```python
from build123d import *
from OCP.BRepFilletAPI import BRepFilletAPI_MakeChamfer

# Parameters (mm, degrees)
SKETCH1_W           = 22.5
SKETCH1_H           = 38
BOSS_EXTRUDE2_DEPTH = 7
SKETCH2_W           = 22.5
SKETCH2_H           = 38
BOSS_EXTRUDE4_DEPTH = 2.5
SKETCH3_W           = 12
SKETCH3_H           = 12
CUT_EXTRUDE1_DEPTH  = 2.5
CHAMFER1_SIZE       = 1.5
FILLET3_R           = 2
FILLET4_R           = 2
CHAMFER2_SIZE       = 3
CHAMFER2_SIZE2      = 1.732050808
FILLET5_R           = 2


with BuildPart() as part:
    # Sketch1 → Boss-Extrude2 (new body)
    with BuildSketch(Plane(origin=(0, 0, 0), x_dir=(1, 0, 0), z_dir=(0, 1, 0))):
        Rectangle(SKETCH1_W, SKETCH1_H)
        Polygon((-8.05, -15.8), (-8.05, -4.492937268), (-10.337901284, -4.492937268), (-10.337901284, 0), (-10.337901284, 4.511829369), (-8.05, 4.511829369), (-8.05, 15.8), (8.05, 15.8), (8.05, 4.494825775), (10.314669875, 4.494825775), (10.314669875, 0), (10.314669875, -4.426605317), (8.05, -4.426605317), (8.05, -15.8), align=None, mode=Mode.SUBTRACT)
    extrude(amount=BOSS_EXTRUDE2_DEPTH)

    # Sketch2 → Boss-Extrude4 (add)
    with BuildSketch(Plane(origin=(0, 7, 0), x_dir=(1, 0, 0), z_dir=(0, 1, 0))):
        Rectangle(SKETCH2_W, SKETCH2_H)
    extrude(amount=BOSS_EXTRUDE4_DEPTH)

    # Sketch3 → Cut-Extrude1 (cut)
    with BuildSketch(Plane(origin=(0, 9.5, 0), x_dir=(1, 0, 0), z_dir=(0, 1, 0))):
        Rectangle(SKETCH3_W, SKETCH3_H)
    extrude(amount=-CUT_EXTRUDE1_DEPTH, mode=Mode.SUBTRACT)

    # Chamfer1
    chamfer1_edges = [part.edges().sort_by_distance(p)[0] for p in [
        (6, 8.25, -6),
        (6, 8.25, 6),
        (-6, 8.25, 6),
        (-6, 8.25, -6),
    ]]
    chamfer(chamfer1_edges, length=CHAMFER1_SIZE)

    # Fillet3
    fillet3_edges = [part.edges().sort_by_distance(p)[0] for p in [
        (8.05, 7, 10.113302659),
        (0, 7, 15.8),
        (-8.05, 7, 10.146468634),
        (-9.193950642, 7, 4.492937268),
        (-8.05, 3.5, 15.8),
        (8.05, 3.5, 15.8),
        (-9.193950642, 7, -4.511829369),
        (-8.05, 7, -10.155914685),
        (0, 7, -15.8),
        (8.05, 7, -10.147412887),
        (9.182334937, 7, -4.494825775),
        (9.182334937, 7, 4.426605317),
    ]]
    fillet(fillet3_edges, radius=FILLET3_R)

    # Fillet4
    # the kernel refuses this fillet: 2 mm, written as the material it adds along each edge
    with BuildSketch(Plane(origin=(-6.05, 5, -13.8), x_dir=(-1, 0, 0), z_dir=(0, 0, -1))) as fillet4_piece_1_section:
        Polygon((0, 0), (FILLET4_R, 0), (FILLET4_R, FILLET4_R), (0, FILLET4_R), align=None)
    fillet4_piece_1 = extrude(amount=FILLET4_R, mode=Mode.PRIVATE)
    fillet4_piece_1 = fillet4_piece_1 - Plane(origin=(-6.05, 5, -13.8), x_dir=(0.7071067811865475, -0.7071067811865475, 0), z_dir=(0, 0, -1)) * Sphere(FILLET4_R, mode=Mode.PRIVATE)
    add(fillet4_piece_1)
    with BuildSketch(Plane(origin=(6.05, 5, -13.8), x_dir=(0, 0, -1), z_dir=(1, 0, 0))) as fillet4_piece_2_section:
        Polygon((0, 0), (FILLET4_R, 0), (FILLET4_R, FILLET4_R), (0, FILLET4_R), align=None)
    fillet4_piece_2 = extrude(amount=FILLET4_R, mode=Mode.PRIVATE)
    fillet4_piece_2 = fillet4_piece_2 - Plane(origin=(6.05, 5, -13.8), x_dir=(0, -0.7071067811865475, 0.7071067811865475), z_dir=(1, 0, 0)) * Sphere(FILLET4_R, mode=Mode.PRIVATE)
    add(fillet4_piece_2)
    with BuildSketch(Plane(origin=(8.05, 0, -15.8), x_dir=(0, 0, 1), z_dir=(0, 1, 0)), Plane(origin=(-8.05, 0, -15.8), x_dir=(1, 0, 0), z_dir=(0, 1, 0))) as fillet4_piece_3:
        with BuildLine():
            CenterArc((FILLET4_R, -FILLET4_R), FILLET4_R, 90, 90)
            Line((0, -FILLET4_R), (0, 0))
            Line((0, 0), (FILLET4_R, 0))
        make_face()
    extrude(amount=5)

    # Chamfer2: one chamfer whose edges measure the first distance from different faces: ONE call of the kernel's chamfer builder (chamfer() names one face for all edges)
    chamfer2_edges_1 = [part.edges().sort_by_distance(p)[0] for p in [
        (11.25, 9.5, 0),
    ]]
    chamfer2_side_1 = [part.faces().sort_by_distance(p)[0] for p in [
        (11.25, 4.75, 0),
    ]]
    chamfer2_edges_2 = [part.edges().sort_by_distance(p)[0] for p in [
        (0, 9.5, -19),
    ]]
    chamfer2_side_2 = [part.faces().sort_by_distance(p)[0] for p in [
        (0, 4.75, -19),
    ]]
    chamfer2_edges_3 = [part.edges().sort_by_distance(p)[0] for p in [
        (-11.25, 9.5, 0),
    ]]
    chamfer2_side_3 = [part.faces().sort_by_distance(p)[0] for p in [
        (-11.25, 4.75, 0),
    ]]
    chamfer2_edges_4 = [part.edges().sort_by_distance(p)[0] for p in [
        (0, 9.5, 19),
    ]]
    chamfer2_side_4 = [part.faces().sort_by_distance(p)[0] for p in [
        (0, 4.75, 19),
    ]]
    chamfer2 = BRepFilletAPI_MakeChamfer(part.part.solid().wrapped)
    for e in chamfer2_edges_1:
        chamfer2.Add(CHAMFER2_SIZE, CHAMFER2_SIZE2, e.wrapped, chamfer2_side_1[0].wrapped)  # the first distance lies on this face
    for e in chamfer2_edges_2:
        chamfer2.Add(CHAMFER2_SIZE, CHAMFER2_SIZE2, e.wrapped, chamfer2_side_2[0].wrapped)  # the first distance lies on this face
    for e in chamfer2_edges_3:
        chamfer2.Add(CHAMFER2_SIZE, CHAMFER2_SIZE2, e.wrapped, chamfer2_side_3[0].wrapped)  # the first distance lies on this face
    for e in chamfer2_edges_4:
        chamfer2.Add(CHAMFER2_SIZE, CHAMFER2_SIZE2, e.wrapped, chamfer2_side_4[0].wrapped)  # the first distance lies on this face
    add(Compound.cast(chamfer2.Shape()), mode=Mode.REPLACE)

    # Fillet5
    fillet5_edges = [part.edges().sort_by_distance(p)[0] for p in [
        (-11.25, 6.5, 0),
        (0, 6.5, -19),
        (11.25, 6.5, 0),
        (0, 6.5, 19),
    ]]
    fillet(fillet5_edges, radius=FILLET5_R)


solid = part.part
```
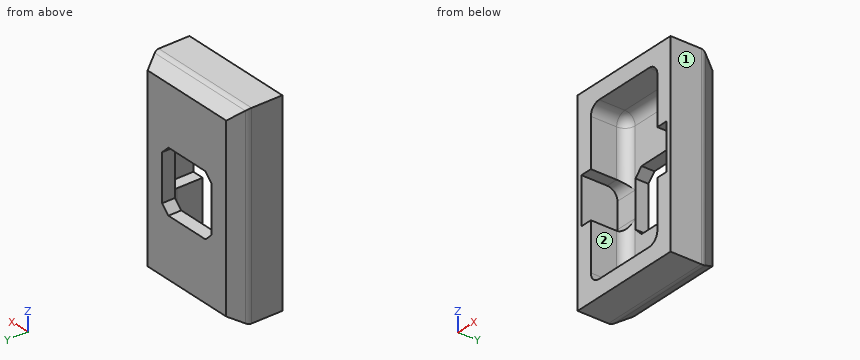
Model file for the job. Use its own axes, mm. Face numbers are marked on the shaded views. A direction names the side the tool comes from. Coordinates: 2 decimals unless noted, no trailing zeros. Write each loop counter-clockwise with the first axis right and the second up, starting at its lowest first coordinate (ties: lowest second). Pieces come first, ordered by that corner, then holes. Notation, with made-up numbers: (27.25, -14.75) - (74.25, -14.75) arc R17 cw to (74.25, -0.75) - close; hole circle Ø10 at (55, 18.25). An arc over 180 degrees is marked (long way). Use a Markdown table: item, result. Add a question column.
Item 1: 3-axis set-ups, long thin cutter, end or side, ignore diameter. For the marked faces 1 and 2: which of +Z, -Z, +X, -X, +Y, -Y reach the whole face in a straight line?
Item 2: Band-saw the part on D-D, the plane x = -8.5. Write the cut outline in (y, z).
Item 3: Band-saw the part on C-C, the plane y = 2. Write the cut outline in (x, z), and give its area (3 significant figures).
Item 4: Band-saw the part on B-B, the plane x = 2.5. Write the cut outline in (y, z).
Item 5: Band-saw the part on A-A, the plane z = -5.5. Write the cut outline in (x, y).
Item 6: Drill centre lines: line 1 along Z through (x, y) = (8.75, 3.5); line 2 along X through (y, z) = (2.75, 1); line 3 along X through (y, z) = (3.75, -9.5). Where is each one in solid material? Low to high.
Item 7: Drop flat-ended pins along their axis: pin 1 (3 mm diameter, centred on x = 0.5, y = 8, fed in from +Z); pin 2 (2 mm diameter, centred on y = 8, z = 0.5, fed in from -X); pin 3 (10.5 mm diameter, centred on x = -3.5, z = 0, fed in from -Y). Give the stop position or say it passes through.
A:
| question | item | result |
|---|---|---|
| 1 | face 1 | +Z, -Z, +X, +Y, -Y |
| 1 | face 2 | -Y |
| 2 | outline | (0, -19) - (5.96, -19) arc R2 ccw to (6.96, -18.73) - (9.5, -17.27) - (9.5, 17.27) - (6.96, 18.73) arc R2 ccw to (5.96, 19) - (0, 19) - (0, 4.49) - (5, 4.49) arc R2 cw to (7, 2.49) - (7, -2.51) arc R2 cw to (5, -4.51) - (0, -4.51) - close |
| 3 | outline | (-11.25, -19) - (11.25, -19) - (11.25, 19) - (-11.25, 19) - close; hole (-10.34, -4.51) - (-8.05, -4.51) - (-8.05, -13.8) arc R2 ccw to (-6.05, -15.8) - (6.05, -15.8) arc R2 ccw to (8.05, -13.8) - (8.05, -4.49) - (10.31, -4.49) - (10.31, 4.43) - (8.05, 4.43) - (8.05, 13.8) arc R2 ccw to (6.05, 15.8) - (-6.05, 15.8) arc R2 ccw to (-8.05, 13.8) - (-8.05, 4.49) - (-10.34, 4.49) - close |
| 3 | area | 309 mm² |
| 4 | outline | (0, -19) - (5.96, -19) arc R2 ccw to (6.96, -18.73) - (9.5, -17.27) - (9.5, -6) - (7, -6) - (7, -13.8) arc R2 cw to (5, -15.8) - (0, -15.8) - close; (0, 15.8) - (5, 15.8) arc R2 cw to (7, 13.8) - (7, 6) - (9.5, 6) - (9.5, 17.27) - (6.96, 18.73) arc R2 ccw to (5.96, 19) - (0, 19) - close |
| 5 | outline | (-11.25, 0) - (-8.05, 0) - (-8.05, 5) arc R2 cw to (-6.05, 7) - (-5, 7) - (-5, 9.5) - (-9.52, 9.5) - (-10.98, 6.96) arc R2 ccw to (-11.25, 5.96) - close; (5, 7) - (6.05, 7) arc R2 cw to (8.05, 5) - (8.05, 0) - (11.25, 0) - (11.25, 5.96) arc R2 ccw to (10.98, 6.96) - (9.52, 9.5) - (5, 9.5) - close |
| 6 | line 1 | z = -19 to -4.49, 4.43 to 19 |
| 6 | line 2 | x = -11.25 to -10.34, 10.31 to 11.25 |
| 6 | line 3 | x = -11.25 to -8.05, 8.05 to 11.25 |
| 7 | pin 1 | stops at z = 18.93 |
| 7 | pin 2 | stops at x = -10.96 |
| 7 | pin 3 | stops at y = 6.61 |
